Geometry: see drawing. Coordinates: mm, zero at the bounding-box minimum. Give positions to 0.01 mm unless a question says otherwise; leave off trailing zeros. Loops run counter-clockwise (first coordinate to the right, second up) from the corner with the lowest first, then second, coordinate; pieces in that order, holes last. Notation, with made-up numbers: (80, -36) - (86, -36) arc R27 cw to (86, -2) - close; hole circle Ø1 at (-29, 4). An arc over 180 degrees is marked (long way). Use one line per item in the form item = value.
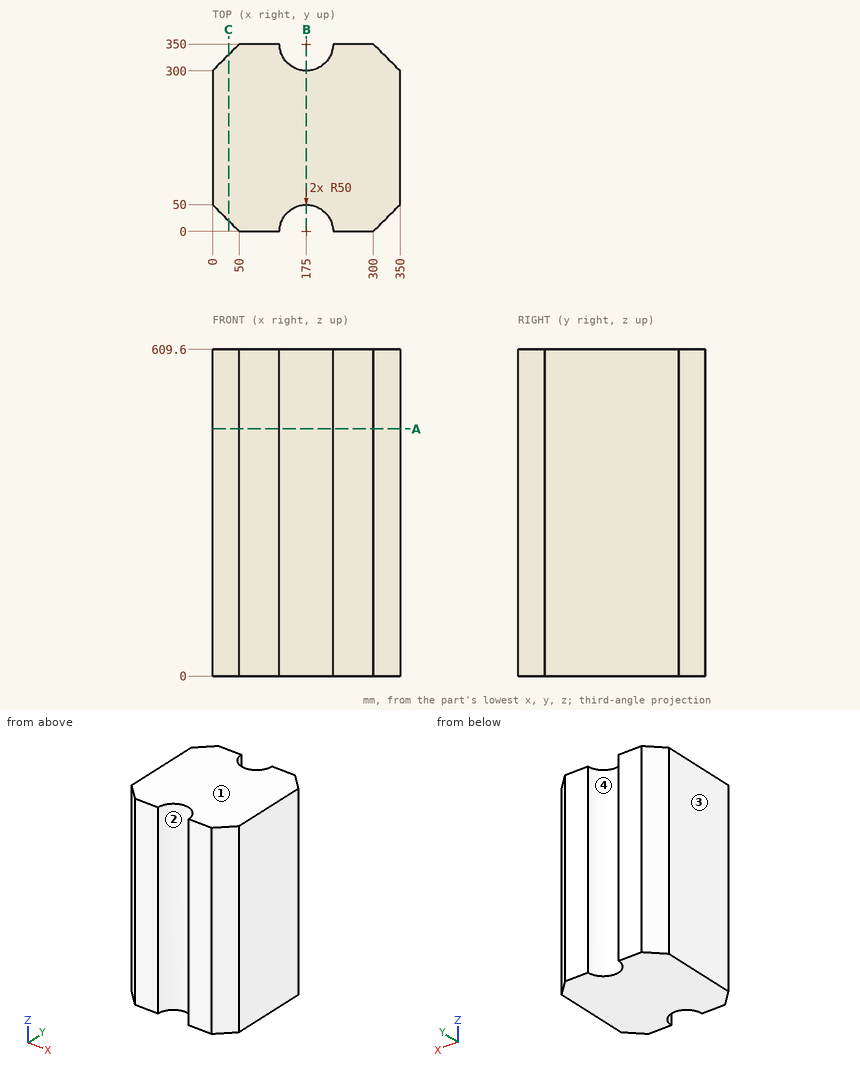
(1) Pin query (flat end, axial travel): P1, Ø5, axis at x = 154, z = 233.5, coming from the +Y side; P2, Ø4, axis at x = 44, z = 255.5, coming from the -Y side. Return the tip coordinate at first contact, or that it passes through.
Solution:
P1 = 305.87
P2 = 4
(2) Cut plane A-A (z = 461.5). Return the cut outline in (x, y).
Solution:
outline = (0, 50) - (50, 0) - (125, 0) arc R50 cw to (225, 0) - (300, 0) - (350, 50) - (350, 300) - (300, 350) - (225, 350) arc R50 cw to (125, 350) - (50, 350) - (0, 300) - close
(3) Pull-direction query (X, two-part tool) for the marked faces 1, 2, 3 and 4; classes: released by +X, released by -X, zero draft, split by the parting line, or undercut.
Solution:
face_1 = zero draft
face_2 = undercut
face_3 = released by -X
face_4 = undercut
(4) Cut plane C-C (x = 30). Return the cut outline in (y, z).
Solution:
outline = (20, 0) - (330, 0) - (330, 609.6) - (20, 609.6) - close
(5) Material intervals for L1, parallel to Y at x = 169, z = 69; L2, parallel to Y at x = 133.5, z = 148, sorted ascending. Write a range as from..to.
Solution:
L1 = 49.64..300.36
L2 = 27.89..322.11
(6) Cut plane B-B (x = 175). Return the cut outline in (y, z), plus the area to 3 significant figures.
Solution:
outline = (50, 0) - (300, 0) - (300, 609.6) - (50, 609.6) - close
area = 152,000 mm2
